Autodesk Inventor part; units mm, degrees
ref_plane "YZ Plane" through (0, 0, 0) normal (1, 0, 0) x (0, 1, 0)
ref_plane "XZ Plane" through (0, 0, 0) normal (0, 1, 0) x (-1, 0, 0)
ref_plane "XY Plane" through (0, 0, 0) normal (0, 0, 1) x (1, 0, 0)
sketch "Sketch1" plane through (0, 0, 0) normal (0, 0, 1) x (1, 0, 0)
  line L0 (0, 0) -> (-84, 0)
  line L1 (-84, 0) -> (-84, -1490)
  line L2 (-84, -1490) -> (0, -1490)
  line L3 (0, -1490) -> (0, 0)
  line L4 (-84, -1390) -> (-40, -1390)
  line L5 (-40, -1390) -> (-40, -1385)
  line L6 (-40, -1385) -> (-84, -1385)
  line L7 (-84, -1385) -> (-84, -1390)
  line L8 (-84, -893.3333) -> (-40, -893.3333)
  line L9 (-40, -893.3333) -> (-40, -888.3333)
  line L10 (-40, -888.3333) -> (-84, -888.3333)
  line L11 (-84, -888.3333) -> (-84, -893.3333)
  line L12 (-84, -396.6667) -> (-40, -396.6667)
  line L13 (-40, -396.6667) -> (-40, -391.6667)
  line L14 (-40, -391.6667) -> (-84, -391.6667)
  line L15 (-84, -391.6667) -> (-84, -396.6667)
  circle A0 centre (-84, -155) radius 30
  line L16 (-84, -953) -> (0, -953)
  line L17 (-84, -155) -> (0, -155)
  point P0 (-84, -391.6667)
  point P1 (-84, -396.6667)
  point P2 (-84, -888.3333)
  point P3 (-84, -893.3333)
  point P4 (-84, -1385)
  point P5 (-84, -125)
  point P6 (-84, -185)
  point P7 (-54, -155)
  dimension "d0" = 1490
  dimension "d1" = 84
  dimension "d2" = 5
  dimension "d4" = 100
  dimension "d7" = 496.6667
  dimension "d23" = 40
  dimension "d28" = 60
  dimension "d29" = 1335
  dimension "d30" = 953
extrude "Plate1" add sketch "Sketch1" along normal blind 4 contours L3 L16 L1 L8 L9 L10 L12 L13 L14 A0 L17
sketch "Sketch2" plane through (-4, -155, 0) normal (1, 0, 0) x (0, 1, 0)
  line L0 (-798, 0) -> (0, 0)
  line L1 (0, 0) -> (0, 60)
  line L2 (0, 60) -> (-798, 60)
  line L3 (-798, 60) -> (-798, 0)
edge flange "Flange1" height 60 angle 90 thickness 4 bend radius 4 thickness toward (1, 0, 0) relief tear relief width 4 relief depth 2 edges at (0, -554, 4) wall of the first edge with corners at (-4, -953, 0) (-4, -155, 0) (-4, -155, 60) (-4, -953, 60)
bend "Bend1"
corner "Corner1"
chamfer "Corner Chamfer1" distance 3 angle 45 4 edges at (-84, -893.3333, 2) (-84, -888.3333, 2) (-84, -391.6667, 2) (-84, -396.6667, 2)
equation "\"d0\" = Стрингер_длина"
equation "\"d2\" = паз_под_стрингер_толщина"
equation "\"d7\" = Шаг_шпангоутов"
equation "\"d28\" = 2 * радиус_выреза_под_сварку"
equation "\"d12\" = Thickness"
equation "\"d13\" = BendReliefWidth"
equation "\"d14\" = BendReliefDepth"
equation "\"d15\" = MinimumRemnant"
equation "\"d16\" = TransitionRadius"
equation "\"d17\" = ребро_усилителей"
equation "\"d19\" = BendRadius"
equation "\"d20\" = CornerReliefSize"
equation "\"d21\" = GapSize"
equation "\"d22\" = JacobiRadiusSize"
equation "\"BendRadius\" = Thickness"
equation "\"BendReliefWidth\" = Thickness"
equation "\"BendReliefDepth\" = 0.5 * Thickness"
equation "\"CornerReliefSize\" = 4 * Thickness"
equation "\"MinimumRemnant\" = 2 * Thickness"
equation "\"TransitionRadius\" = BendRadius"
equation "\"JacobiRadiusSize\" = BendRadius"
equation "\"GapSize\" = Thickness"
properties part number "GBK 0104 stringer 3_Dummy" material "Steel"
Model file for the job. Use its own axes, mm. A direction names the side the tool comes from. Give positions to 0.01 mm unless a question says otherwise; leave off trailing zeros. Write each loop counter-clockwise with the first axis right and the second up, starting at its lowest first coordinate (ties: lowest second). Pieces come first, ordered by that corner, then holes. Notation, with made-up numbers: M -20,50 L -15,50 A35 ccw -15,84 Z; hole C -24,38.25 d3. An arc over 180 degrees is marked long. Use a Markdown table: item, result.
1) Cut at A-A (y = -790). List the corners of the cut face in (x, z), and give its area (3 significant figures).
Responses:
| item | result |
|---|---|
| outline | M -84,0 L -8,0 A8 ccw 0,8 L 0,60 L -4,60 L -4,8 A4 cw -8,4 L -84,4 Z |
| area | 550 mm2 |
2) Pin check, flat tips, straight feed: pin 1 (4.5 mm diameter, centred on y = -891, z = 3, fed in from -X); pin 2 (15.5 mm diameter, centred on y = -614, z = 27.5, fed in from -X); pin 3 (10 mm diameter, centred on x = -11, y = -299, fed in from +Z); pin 4 (2 mm diameter, centred on y = -350, z = 31.5, fed in from +X). Stop position of each tip, or through.
Responses:
| item | result |
|---|---|
| pin 1 | stops at x = -40 |
| pin 2 | stops at x = -4 |
| pin 3 | stops at z = 4.54 |
| pin 4 | stops at x = 0 |
3) Cut at C-C (x = -29.5). List the corners of the cut face in (y, z).
Responses:
| item | result |
|---|---|
| outline | M -953,0 L -155,0 L -155,4 L -953,4 Z |
4) Cut at B-B (z = 18). List the corners of the cut face in (x, y).
Responses:
| item | result |
|---|---|
| outline | M -4,-953 L 0,-953 L 0,-155 L -4,-155 Z |
5) Tool access for faces 1 (the flat face through (-3, -155, 17)), 2 (the flat face through (-47, -548, 4)): list every direction of +Z, -Z, +X, -X, +Y, -Y with a clear straight run to the whole face (end or side of a thin tool).
Responses:
| item | result |
|---|---|
| face 1 | +Z, -Z, +X, -X, +Y |
| face 2 | +Z, -X, +Y, -Y |
6) Drill centre lines: line 1 (X direction, y = -723, z = 33); line 2 (Z direction, x = -70.5, y = -281); line 3 (Y direction, x = -71, z = 3). Where is each one in solid material? Low to high. Write a range as from..to.
Responses:
| item | result |
|---|---|
| line 1 | x = -4..0 |
| line 2 | z = 0..4 |
| line 3 | y = -953..-893.33, -888.33..-396.67, -391.67..-182.04 |
